Source: CAD feature listing. Evaluate the final solid. Frame: model axes, mm. Face numbers are marked on the shaded views. A direction names the side the tool comes from. Round coordinates to 2 decimals unless told otherwise and drop trailing zeros. Write each loop counter-clockwise with the first axis right and the second up, starting at its lowest first coordinate (ties: lowest second). Pieces come first, ordered by that corner, then holes. Notation, with made-up numbers: M 81.5,36.25 L 104.5,36.25 A35 cw 104.5,69.25 Z; hole C 42,61 d7. An arc over 180 degrees is marked long. Answer in a Markdown table with one row per item.
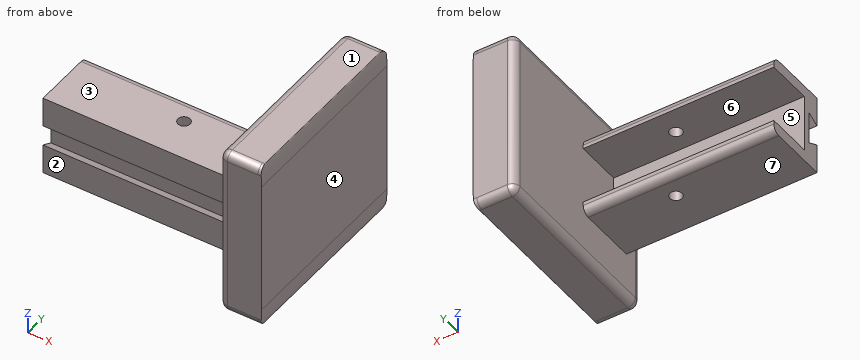
from build123d import *

# Parameters (mm, degrees)
EXTRUDE_1_OUTLINE_W = 50
EXTRUDE_1_OUTLINE_H = 5
EXTRUDE_1_DEPTH     = 21.2
SKETCH_3_W          = 45
SKETCH_3_H          = 49.4
EXTRUDE_1_2_DEPTH   = 10
CUT_EXTRUDE_1_DEPTH = 57
SKETCH_5_W          = 50
SKETCH_5_H          = 3
EXTRUDE_2_DEPTH     = 12
SKETCH_8_R          = 1.6
CUT_EXTRUDE_2_DEPTH = 95.509364615
FILLET_1_R          = 2
SKETCH_9_W          = 45
SKETCH_9_H          = 49.4
EXTRUDE_3_DEPTH     = 1
FILLET_2_R          = 2
FILLET_3_SIZE       = 5
FILLET_3_SIZE_2     = 0.5


with BuildPart() as part:
    # Extrude 1: read off the stored shape, not the designer's step
    # Extrude 1 outline → Extrude 1 (new body)
    with BuildSketch(Plane.XY):
        with Locations((45, -3.5)):
            Rectangle(EXTRUDE_1_OUTLINE_W, EXTRUDE_1_OUTLINE_H)
    extrude(amount=EXTRUDE_1_DEPTH)

    # 草图3 → Extrude 1 2 (add)
    with BuildSketch(Plane(origin=(70, 0, 0), x_dir=(0, 0, -1), z_dir=(1, 0, 0))):
        with Locations((-10.6, 13.2)):
            Rectangle(SKETCH_3_W, SKETCH_3_H)
    extrude(amount=EXTRUDE_1_2_DEPTH)

    # 草图4 → 切除-拉伸1 (cut)
    with BuildSketch(Plane.ZY.offset(-20)):
        Polygon((10.6, -6), (13.325, -6), (14.875, -2.9), (6.325, -2.9), (7.875, -6), align=None)
    extrude(amount=-CUT_EXTRUDE_1_DEPTH, mode=Mode.SUBTRACT)

    # 草图5 → 凸台-拉伸2 (add)
    with BuildSketch(Plane(origin=(0, -1, 0), x_dir=(1, 0, 0), z_dir=(0, 1, 0))):
        with Locations((45, -1.5)):
            Rectangle(SKETCH_5_W, SKETCH_5_H)
        with Locations((45, -19.7)):
            Rectangle(SKETCH_5_W, SKETCH_5_H)
    extrude(amount=EXTRUDE_2_DEPTH)

    # 草图8 → 切除-拉伸2 (cut, through all)
    with BuildSketch(Plane.XY.offset(21.2)):
        with Locations((50, 4.5)):
            Circle(SKETCH_8_R)
    extrude(amount=-CUT_EXTRUDE_2_DEPTH, mode=Mode.SUBTRACT)

    # 圆角1
    fillet_1_edges = [part.edges().sort_by_distance(p)[0] for p in [
        (70, 13.2, 33.1),
        (75, 37.9, 33.1),
        (70, -11.5, 10.6),
        (75, -11.5, 33.1),
        (70, 13.2, -11.9),
        (75, -11.5, -11.9),
        (70, 37.9, 10.6),
        (75, 37.9, -11.9),
        (45, 11, 0),
        (45, 11, 21.2),
    ]]
    fillet(fillet_1_edges, radius=FILLET_1_R)

    # 草图9 → 凸台-拉伸3 (add)
    with BuildSketch(Plane(origin=(80, 0, 0), x_dir=(0, 0, -1), z_dir=(1, 0, 0))):
        with Locations((-10.6, 13.2)):
            Rectangle(SKETCH_9_W, SKETCH_9_H)
    extrude(amount=EXTRUDE_3_DEPTH)

    # 圆角2
    fillet_2_edges = [part.edges().sort_by_distance(p)[0] for p in [
        (80.5, 37.9, 33.1),
        (80.5, -11.5, 33.1),
        (80.5, -11.5, -11.9),
        (80.5, 37.9, -11.9),
    ]]
    fillet(fillet_2_edges, radius=FILLET_2_R)

    # 圆角3
    # a fillet whose section is not a circle: 5, 0.5 mm, written as the material it takes off along each edge
    with BuildSketch(Plane(origin=(81, 48.4, -11.9), x_dir=(0, 0, 1), z_dir=(0, -1, 0)), Plane(origin=(81, -22, 33.1), x_dir=(0, 0, -1), z_dir=(0, 1, 0))) as fillet_3_piece_1:
        with BuildLine():
            Bezier((FILLET_3_SIZE, 0), (0, 0), (0, FILLET_3_SIZE_2), weights=[1, 0.707106781, 1])
            Line((0, FILLET_3_SIZE_2), (0, 0))
            Line((0, 0), (FILLET_3_SIZE, 0))
        make_face()
    extrude(amount=70.4, mode=Mode.SUBTRACT)


solid = part.part
Q1. Section D-D (x = 40). Return loops of the section in (y, z) (3 decimals), and give its area (3 significant figures).
Solutions:
| item | result |
|---|---|
| outline | M -6,0 L 9,0 A2 ccw 11,2 L 11,3 L -1,3 L -1,18.2 L 11,18.2 L 11,19.2 A2 ccw 9,21.2 L -6,21.2 L -6,13.325 L -2.9,14.875 L -2.9,6.325 L -6,7.875 Z |
| area | 155 mm2 |
Q2. Section B-B (z = 9.5). Return loops of the section in (x, y).
Solutions:
| item | result |
|---|---|
| outline | M 20,-2.9 L 77,-2.9 L 77,-6 L 70,-6 L 70,-9.5 A2 ccw 72,-11.5 L 81,-11.5 L 81,37.9 L 72,37.9 A2 ccw 70,35.9 L 70,-1 L 20,-1 Z |
Q3. Pull-direction query (Z, two-part tool) for the marked faces 4, 5, 6 and 7; classes: pulls with the +Z half, pulls with the -Z half, needs draft (parallel to the pull), parting line crosses it, or undercut.
Solutions:
| item | result |
|---|---|
| face 4 | needs draft |
| face 5 | undercut |
| face 6 | undercut |
| face 7 | pulls with the -Z half |
Q4. Section C-C (y = 4.5). State how many separate pieces and enclosed holes the cut face has, and give its area (3 significant figures).
Solutions:
| item | result |
|---|---|
| separate pieces | 3 |
| enclosed holes | 0 |
| area | 773 mm2 |
Q5. Access query for the marked faces 1, 2 and 3. Directions: +Z, -Z, +X, -X, +Y, -Y. A direction counts if a zero-diameter tool reaches every point of the face in a straight line with its end or side. Return the directions, or none.
Solutions:
| item | result |
|---|---|
| face 1 | +Z, +X, -X, +Y, -Y |
| face 2 | +Z, -Z, -X, -Y |
| face 3 | +Z, -X, +Y, -Y |
Q6. Material intervals for probe 1 along Z at (x, y) = (64, 2.5); probe 2 along X at (y, z) = (18, -7); probe 3 along Y at (x, z) = (50, 1.85), sorted ascending.
Solutions:
| item | result |
|---|---|
| probe 1 | z = 0 to 3, 18.2 to 21.2 |
| probe 2 | x = 70 to 81 |
| probe 3 | y = -6 to 2.9, 6.1 to 10.99 |
Q7. Contact query for flat-ended pins moving along their axis: pin 1 Ø3.5 at (x, y) = (40.5, 6) entering from +Z; pin 2 Ø20.5 at (y, z) = (22.5, 14.5) entering from -X; pin 3 Ø12 at (x, y) = (42, 5) entering from -Z. Output: stop coordinate, or through.
Solutions:
| item | result |
|---|---|
| pin 1 | stops at z = 21.2 |
| pin 2 | stops at x = 70 |
| pin 3 | stops at z = 0 |
Q8. Section A-A (x = 50). Return loops of the section in (y, z) (3 decimals).
Solutions:
| item | result |
|---|---|
| outline | M -6,0 L 2.9,0 L 2.9,3 L -1,3 L -1,18.2 L 2.9,18.2 L 2.9,21.2 L -6,21.2 L -6,13.325 L -2.9,14.875 L -2.9,6.325 L -6,7.875 Z; M 6.1,0 L 9,0 A2 ccw 11,2 L 11,3 L 6.1,3 Z; M 6.1,18.2 L 11,18.2 L 11,19.2 A2 ccw 9,21.2 L 6.1,21.2 Z |
